Check sheet for the modelled part. Datum: model origin and axes. Units: mm. A direction names the side the tool comes from. Round coordinates to 2 decimals unless told otherwise and drop trailing zeros. Write each loop counter-clockwise with the first axis right and the second up, starting at its lowest first coordinate (ties: lowest second). Pieces come first, ordered by that corner, then holes. Notation, with made-up numbers: (1.5, 73.25) -> (58.5, 73.25) arc R31 ccw to (58.5, 102.25) -> close; hole circle Ø5 at (10, 56.25). An arc over 180 degrees is marked (long way). One line per item, written item: value.
Autodesk Inventor part; units mm, degrees
ref_plane "YZ Plane" through (0, 0, 0) normal (1, 0, 0) x (0, 1, 0)
ref_plane "XZ Plane" through (0, 0, 0) normal (0, 1, 0) x (-1, 0, 0)
ref_plane "XY Plane" through (0, 0, 0) normal (0, 0, 1) x (1, 0, 0)
sketch "Náčrt1" plane through (0, 0, 0) normal (0, 0, 1) x (1, 0, 0)
  line L0 (-100, -100) -> (100, -100)
  line L1 (100, -100) -> (100, 100)
  line L2 (100, 100) -> (-100, 100)
  line L3 (-100, 100) -> (-100, -100)
  line L4 (-100, -100) -> (100, 100) construction
  line L5 (100, -100) -> (-100, 100) construction
  point P0 (0, 0)
  dimension "d0" = 200
extrude "Vysunutí1" add sketch "Náčrt1" along normal blind 700
sketch "Náčrt2" plane through (0, 0, 0) normal (1, 0, 0) x (0, 1, 0)
  line L0 (-100, 0) -> (-100, 700)
  line L1 (-150, 760) -> (-150, 1045)
  line L2 (-120, 681.7157) -> (-120, 540)
  line L3 (-100, 700) -> (100, 700)
  line L4 (0, 700) -> (0, 773.8359) construction
  line L5 (-100, 0) -> (100, 0)
  line L6 (-100, 540) -> (-100, 710)
  line L7 (-100, 710) -> (-150, 760)
  line L8 (-170, 1045) -> (-170, 751.7157)
  line L9 (-170, 751.7157) -> (-120, 701.7157)
  line L10 (-120, 701.7157) -> (-120, 540)
  line L11 (-170, 1045) -> (-150, 1045)
  line L12 (-120, 540) -> (-100, 540)
  line L13 (-170, 1010) -> (-150, 1010) construction
  point P0 (0, 0)
  dimension "d5" = 150
  dimension "d22" = 135
  dimension "d24" = 20
  dimension "d26" = 10
  dimension "d35" = 345
  dimension "d36" = 35
extrude "Vysunutí2" add sketch "Náčrt2" along normal mid plane 70
sketch "Náčrt3" plane through (-30, -170, 712.0978) normal (0, -1, 0) x (1, 0, 0)
  line L0 (-5, 332.9022) -> (65, 332.9022)
  line L1 (30, 332.9022) -> (30, 269.5637) construction
  circle A0 centre (30, 297.9022) radius 20
  point P0 (30, -712.0978)
  dimension "d11" = 40
  dimension "d12" = 35
  dimension "d25" = 70
extrude "Vysunutí3" cut sketch "Náčrt3" against normal blind 60
chamfer "Zkosení1" distance 10 angle 45 2 edges at (35, -160, 1045) (-35, -160, 1045)
mirror "Zrcadlit1" about plane through (0, 0, 0) normal (0, 1, 0)
sketch "Náčrt4" plane through (-100, -100, 0) normal (0, -1, 0) x (1, 0, 0)
  circle A0 centre (100, 1010) radius 20
  circle A1 centre (100, 60) radius 20
  line L0 (0, 0) -> (200, 0)
  line L1 (100, 0) -> (100, 549.2134) construction
  dimension "d27" = 40
  dimension "d28" = 60
  dimension "d29" = 950
extrude "Vysunutí4" cut sketch "Náčrt4" against normal through all contours A1
chamfer "Zkosení2" distance 50 angle 45 1 edges at (100, 0, 0)
equation "\"d12\" = 0.5 * d25"
properties part number "B5-A1"
Item 1: Sectioned sample at D-D on y = 84. Enter the section's corners in (x, z).
Answer:
outline: (-100, 0) -> (50, 0) -> (100, 50) -> (100, 700) -> (-100, 700) -> close; hole circle Ø40 at (0, 60)
Item 2: Mould release check, pull along Z, two halves, no side actions. Record for faces 1 (the flat face through (0, 110, 540)), 2 (the cylindrical face through (10.752, -160.14, 1026.864)), 3 (the flat face through (0, -120, 622)): pulls with the +Z half, pulls with the -Z half, needs draft (parallel to the pull), parting line crosses it, or undercut.
Answer:
face 1: pulls with the -Z half
face 2: undercut
face 3: needs draft
Item 3: Sectioned sample at C-C on z = 1010. Enter the section's corners in (x, y), and give its area (3 significant figures).
Answer:
outline: (-35, -170) -> (-20, -170) -> (-20, -150) -> (-35, -150) -> close; (-35, 150) -> (-20, 150) -> (-20, 170) -> (-35, 170) -> close; (20, -170) -> (35, -170) -> (35, -150) -> (20, -150) -> close; (20, 150) -> (35, 150) -> (35, 170) -> (20, 170) -> close
area: 1,200 mm^2
Item 4: Sectioned sample at A-A on z = 866. Enter the section's corners in (x, y).
Answer:
outline: (-35, -170) -> (35, -170) -> (35, -150) -> (-35, -150) -> close; (-35, 150) -> (35, 150) -> (35, 170) -> (-35, 170) -> close
Item 5: Depth check by flat-ended pin: P1, Ø5, axis at x = 20.5, y = -42.5, coming from the +Z side; P2, Ø5, axis at x = 8.5, z = 704, coming from the +Y side; P3, Ø12, axis at x = -9, y = -10, coming from the -Z side; P4, Ø1.5, axis at x = -25.5, z = 479.5, coming from the -Y side. Enter the tip coordinate at first touch or a pass-through.
Answer:
P1: stops at z = 700
P2: stops at y = 124.78
P3: stops at z = 0
P4: stops at y = -100
Item 6: Tool access check on faces 4 (the flat face through (35, 153, 789)), 5 (the flat face through (0, -125, 735)), 6 (the flat face through (0, 120, 620)). Record the directions out of +Z, -Z, +X, -X, +Y, -Y that give a thin tool (end or side, any length) a straight path to the whole face; none if there is none.
Answer:
face 4: +Z, -Z, +X, +Y
face 5: +Z, +X, -X
face 6: -Z, +X, -X, +Y
Item 7: Thickness scan on line 1 (Y direction, x = 11.5, z = 894.5); line 2 (Z direction, x = 33.5, y = -28.5); line 3 (Y direction, x = -38, z = 590). Record the ranges inside material, lowest first.
Answer:
line 1: y = -170 to -150, 150 to 170
line 2: z = 0 to 700
line 3: y = -100 to 100
Item 8: Sectioned sample at B-B on x = 0. Count the separate pieces of the cut face and the enclosed holes in it, and give its area (3 significant figures).
Answer:
separate pieces: 4
enclosed holes: 0
area: 151,000 mm^2
